Work out the finished part from the listing and answer in its coordinate system (mm). Give positions to 0.01 mm unless a question says otherwise; leave off trailing zeros. One line per item, written item: value.
from build123d import *

# Parameters (mm, degrees)
SKETCH1_R      = 3.4036
EXTRUDE1_DEPTH = 317.5


with BuildPart() as part:
    # Sketch1 → Extrude1 (new, symmetric)
    with BuildSketch(Plane.XY):
        with BuildLine():
            Line((-19.939, 16.891), (-19.939, 4.7625))
            ThreePointArc((-19.939, 4.7625), (-19.715815367, 4.223684633), (-19.177, 4.0005))
            Line((-19.177, 4.0005), (-16.2052, 4.0005))
            ThreePointArc((-16.2052, 4.0005), (-15.666384633, 4.223684633), (-15.4432, 4.7625))
            Line((-15.4432, 4.7625), (-15.4432, 10.424558599))
            ThreePointArc((-15.4432, 10.424558599), (-14.972804775, 11.128554802), (-14.142384633, 10.963373966))
            Line((-14.142384633, 10.963373966), (-8.574059555, 5.395048889))
            ThreePointArc((-8.574059555, 5.395048889), (-7.924348265, 4.422687227), (-7.6962, 3.275708444))
            Line((-7.6962, 3.275708444), (-7.6962, -3.275708444))
            ThreePointArc((-7.6962, -3.275708444), (-7.924348265, -4.422687227), (-8.574059555, -5.395048889))
            Line((-8.574059555, -5.395048889), (-14.142384633, -10.963373966))
            ThreePointArc((-14.142384633, -10.963373966), (-14.972804775, -11.128554802), (-15.4432, -10.424558599))
            Line((-15.4432, -10.424558599), (-15.4432, -4.7625))
            ThreePointArc((-15.4432, -4.7625), (-15.666384633, -4.223684633), (-16.2052, -4.0005))
            Line((-16.2052, -4.0005), (-19.177, -4.0005))
            ThreePointArc((-19.177, -4.0005), (-19.715815367, -4.223684633), (-19.939, -4.7625))
            Line((-19.939, -4.7625), (-19.939, -16.891))
            ThreePointArc((-19.939, -16.891), (-19.046261469, -19.046261469), (-16.891, -19.939))
            Line((-16.891, -19.939), (-4.7625, -19.939))
            ThreePointArc((-4.7625, -19.939), (-4.223684633, -19.715815367), (-4.0005, -19.177))
            Line((-4.0005, -19.177), (-4.0005, -16.2052))
            ThreePointArc((-4.0005, -16.2052), (-4.223684633, -15.666384633), (-4.7625, -15.4432))
            Line((-4.7625, -15.4432), (-10.424558599, -15.4432))
            ThreePointArc((-10.424558599, -15.4432), (-11.128554802, -14.972804775), (-10.963373966, -14.142384633))
            Line((-10.963373966, -14.142384633), (-5.395048889, -8.574059555))
            ThreePointArc((-5.395048889, -8.574059555), (-4.422687227, -7.924348265), (-3.275708444, -7.6962))
            Line((-3.275708444, -7.6962), (3.275708444, -7.6962))
            ThreePointArc((3.275708444, -7.6962), (4.422687227, -7.924348265), (5.395048889, -8.574059555))
            Line((5.395048889, -8.574059555), (10.963373966, -14.142384633))
            ThreePointArc((10.963373966, -14.142384633), (11.128554802, -14.972804775), (10.424558599, -15.4432))
            Line((10.424558599, -15.4432), (4.7625, -15.4432))
            ThreePointArc((4.7625, -15.4432), (4.223684633, -15.666384633), (4.0005, -16.2052))
            Line((4.0005, -16.2052), (4.0005, -19.177))
            ThreePointArc((4.0005, -19.177), (4.223684633, -19.715815367), (4.7625, -19.939))
            Line((4.7625, -19.939), (19.939, -19.939))
            Line((19.939, -19.939), (35.1155, -19.939))
            ThreePointArc((35.1155, -19.939), (35.654315367, -19.715815367), (35.8775, -19.177))
            Line((35.8775, -19.177), (35.8775, -16.2052))
            ThreePointArc((35.8775, -16.2052), (35.654315367, -15.666384633), (35.1155, -15.4432))
            Line((35.1155, -15.4432), (29.453441401, -15.4432))
            ThreePointArc((29.453441401, -15.4432), (28.749445198, -14.972804775), (28.914626034, -14.142384633))
            Line((28.914626034, -14.142384633), (34.482951111, -8.574059555))
            ThreePointArc((34.482951111, -8.574059555), (35.455312773, -7.924348265), (36.602291556, -7.6962))
            Line((36.602291556, -7.6962), (43.153708444, -7.6962))
            ThreePointArc((43.153708444, -7.6962), (44.300687227, -7.924348265), (45.273048889, -8.574059555))
            Line((45.273048889, -8.574059555), (50.841373966, -14.142384633))
            ThreePointArc((50.841373966, -14.142384633), (51.006554802, -14.972804775), (50.302558599, -15.4432))
            Line((50.302558599, -15.4432), (44.6405, -15.4432))
            ThreePointArc((44.6405, -15.4432), (44.101684633, -15.666384633), (43.8785, -16.2052))
            Line((43.8785, -16.2052), (43.8785, -19.177))
            ThreePointArc((43.8785, -19.177), (44.101684633, -19.715815367), (44.6405, -19.939))
            Line((44.6405, -19.939), (56.769, -19.939))
            ThreePointArc((56.769, -19.939), (58.924261469, -19.046261469), (59.817, -16.891))
            Line((59.817, -16.891), (59.817, -4.7625))
            ThreePointArc((59.817, -4.7625), (59.593815367, -4.223684633), (59.055, -4.0005))
            Line((59.055, -4.0005), (56.0832, -4.0005))
            ThreePointArc((56.0832, -4.0005), (55.544384633, -4.223684633), (55.3212, -4.7625))
            Line((55.3212, -4.7625), (55.3212, -10.424558599))
            ThreePointArc((55.3212, -10.424558599), (54.850804775, -11.128554802), (54.020384633, -10.963373966))
            Line((54.020384633, -10.963373966), (48.452059555, -5.395048889))
            ThreePointArc((48.452059555, -5.395048889), (47.802348265, -4.422687227), (47.5742, -3.275708444))
            Line((47.5742, -3.275708444), (47.5742, 3.275708444))
            ThreePointArc((47.5742, 3.275708444), (47.802348265, 4.422687227), (48.452059555, 5.395048889))
            Line((48.452059555, 5.395048889), (54.020384633, 10.963373966))
            ThreePointArc((54.020384633, 10.963373966), (54.850804775, 11.128554802), (55.3212, 10.424558599))
            Line((55.3212, 10.424558599), (55.3212, 4.7625))
            ThreePointArc((55.3212, 4.7625), (55.544384633, 4.223684633), (56.0832, 4.0005))
            Line((56.0832, 4.0005), (59.055, 4.0005))
            ThreePointArc((59.055, 4.0005), (59.593815367, 4.223684633), (59.817, 4.7625))
            Line((59.817, 4.7625), (59.817, 16.891))
            ThreePointArc((59.817, 16.891), (58.924261469, 19.046261469), (56.769, 19.939))
            Line((56.769, 19.939), (44.6405, 19.939))
            ThreePointArc((44.6405, 19.939), (44.101684633, 19.715815367), (43.8785, 19.177))
            Line((43.8785, 19.177), (43.8785, 16.2052))
            ThreePointArc((43.8785, 16.2052), (44.101684633, 15.666384633), (44.6405, 15.4432))
            Line((44.6405, 15.4432), (50.302558599, 15.4432))
            ThreePointArc((50.302558599, 15.4432), (51.006554802, 14.972804775), (50.841373966, 14.142384633))
            Line((50.841373966, 14.142384633), (45.273048889, 8.574059555))
            ThreePointArc((45.273048889, 8.574059555), (44.300687227, 7.924348265), (43.153708444, 7.6962))
            Line((43.153708444, 7.6962), (36.602291556, 7.6962))
            ThreePointArc((36.602291556, 7.6962), (35.455312773, 7.924348265), (34.482951111, 8.574059555))
            Line((34.482951111, 8.574059555), (28.914626034, 14.142384633))
            ThreePointArc((28.914626034, 14.142384633), (28.749445198, 14.972804775), (29.453441401, 15.4432))
            Line((29.453441401, 15.4432), (35.1155, 15.4432))
            ThreePointArc((35.1155, 15.4432), (35.654315367, 15.666384633), (35.8775, 16.2052))
            Line((35.8775, 16.2052), (35.8775, 19.177))
            ThreePointArc((35.8775, 19.177), (35.654315367, 19.715815367), (35.1155, 19.939))
            Line((35.1155, 19.939), (4.7625, 19.939))
            ThreePointArc((4.7625, 19.939), (4.223684633, 19.715815367), (4.0005, 19.177))
            Line((4.0005, 19.177), (4.0005, 16.2052))
            ThreePointArc((4.0005, 16.2052), (4.223684633, 15.666384633), (4.7625, 15.4432))
            Line((4.7625, 15.4432), (10.424558599, 15.4432))
            ThreePointArc((10.424558599, 15.4432), (11.128554802, 14.972804775), (10.963373966, 14.142384633))
            Line((10.963373966, 14.142384633), (5.395048889, 8.574059555))
            ThreePointArc((5.395048889, 8.574059555), (4.422687227, 7.924348265), (3.275708444, 7.6962))
            Line((3.275708444, 7.6962), (-3.275708444, 7.6962))
            ThreePointArc((-3.275708444, 7.6962), (-4.422687227, 7.924348265), (-5.395048889, 8.574059555))
            Line((-5.395048889, 8.574059555), (-10.963373966, 14.142384633))
            ThreePointArc((-10.963373966, 14.142384633), (-11.128554802, 14.972804775), (-10.424558599, 15.4432))
            Line((-10.424558599, 15.4432), (-4.7625, 15.4432))
            ThreePointArc((-4.7625, 15.4432), (-4.223684633, 15.666384633), (-4.0005, 16.2052))
            Line((-4.0005, 16.2052), (-4.0005, 19.177))
            ThreePointArc((-4.0005, 19.177), (-4.223684633, 19.715815367), (-4.7625, 19.939))
            Line((-4.7625, 19.939), (-16.891, 19.939))
            ThreePointArc((-16.891, 19.939), (-19.046261469, 19.046261469), (-19.939, 16.891))
        make_face()
        with Locations(Location((0, 0, 0), (0, 0, 180))):
            Circle(SKETCH1_R, mode=Mode.SUBTRACT)
        with Locations(Location((39.878, 0, 0), (0, 0, 180))):
            Circle(SKETCH1_R, mode=Mode.SUBTRACT)
        with BuildLine():
            Line((7.6962, 3.275708444), (7.6962, -3.275708444))
            ThreePointArc((7.6962, -3.275708444), (7.924348265, -4.422687227), (8.574059555, -5.395048889))
            Line((8.574059555, -5.395048889), (17.6911, -14.512089333))
            ThreePointArc((17.6911, -14.512089333), (19.939, -15.4432), (22.1869, -14.512089333))
            Line((22.1869, -14.512089333), (31.303940445, -5.395048889))
            ThreePointArc((31.303940445, -5.395048889), (31.953651735, -4.422687227), (32.1818, -3.275708444))
            Line((32.1818, -3.275708444), (32.1818, 3.275708444))
            ThreePointArc((32.1818, 3.275708444), (31.953651735, 4.422687227), (31.303940445, 5.395048889))
            Line((31.303940445, 5.395048889), (22.1869, 14.512089333))
            ThreePointArc((22.1869, 14.512089333), (19.939, 15.4432), (17.6911, 14.512089333))
            Line((17.6911, 14.512089333), (8.574059555, 5.395048889))
            ThreePointArc((8.574059555, 5.395048889), (7.924348265, 4.422687227), (7.6962, 3.275708444))
        make_face(mode=Mode.SUBTRACT)
    extrude(amount=EXTRUDE1_DEPTH, both=True)


solid = part.part
1. Flat-ended cylindrical pins translate along their axes: pin 1 Ø4 at (x, z) = (43.5, -143) entering from -Y; pin 2 Ø5 at (y, z) = (-0.5, 108) entering from +X; pin 3 Ø3 at (x, y) = (-1.5, 13.5) entering from -Z. Find the tip coordinate at first contact, or state that the pin passes through.
Output:
pin 1: stops at y = -19.94
pin 2: stops at x = 47.57
pin 3: passes through
2. Section A-A (z = 23.5) is taken. Count the separate pieces of the cut face and the enclosed holes in it, and give its area (3 significant figures).
Output:
separate pieces: 1
enclosed holes: 3
area: 1,600 mm²
3. Find the intervals of material crossed by line 1 along Y through (x, z) = (5.5, 2); line 2 along Y through (x, z) = (0, -130); line 3 along X through (y, z) = (7, -75), in increasing order.
Output:
line 1: y = -19.94 to -15.44, -8.68 to 8.68, 15.44 to 19.94
line 2: y = -7.7 to -3.4, 3.4 to 7.7
line 3: x = -19.94 to -15.44, -10.18 to 10.18, 29.7 to 50.06, 55.32 to 59.82
